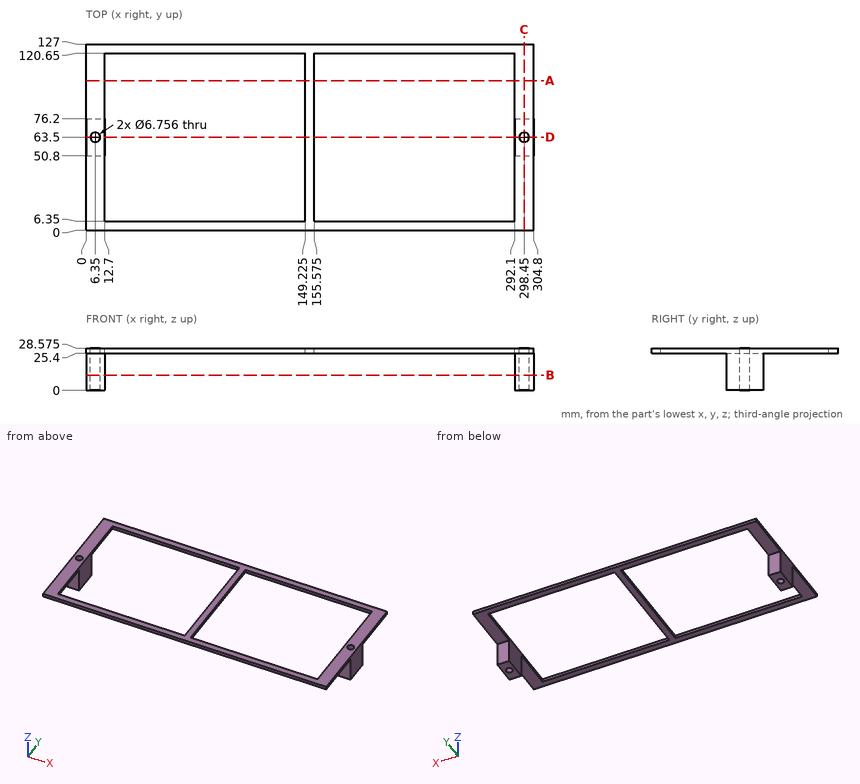
Geometry check sheet. Reference: drawing and pictorial views, mm from the part's lowest x, y, z. Round coordinates to 2 decimals unless told otherwise and drop trailing zeros. Loops run counter-clockwise (first coordinate to the right, second up) from the corner with the lowest first, then second, coordinate; pieces in that order, holes last. Notation, with made-up numbers: (6, -9.5) -> (15, -9.5) arc R17 ccw to (15, -1.5) -> close; hole circle Ø6 at (-10.5, 1.5). An arc over 180 degrees is marked (long way). Use a Markdown table: item, result.
(1) Sectioned sample at D-D (y = 63.5). Enter the section's corners in (x, z) (1 decimal).
Calculated:
| item | result |
|---|---|
| outline | (0, 0) -> (3, 0) -> (3, 28.6) -> (0, 28.6) -> close; (9.7, 0) -> (12.7, 0) -> (12.7, 28.6) -> (9.7, 28.6) -> close; (149.2, 25.4) -> (155.6, 25.4) -> (155.6, 28.6) -> (149.2, 28.6) -> close; (292.1, 0) -> (295.1, 0) -> (295.1, 28.6) -> (292.1, 28.6) -> close; (301.8, 0) -> (304.8, 0) -> (304.8, 28.6) -> (301.8, 28.6) -> close |
(2) Scan lines: probe 1 along X at (y, z) = (63.5, 11); probe 2 along Y at (x, z) = (298.45, 8.5); probe 3 along Y at (x, z) = (180.5, 27.75). Record each from-to range of solid material in increasing order.
Calculated:
| item | result |
|---|---|
| probe 1 | 0 to 2.97, 9.73 to 12.7, 292.1 to 295.07, 301.83 to 304.8 |
| probe 2 | 50.8 to 60.12, 66.88 to 76.2 |
| probe 3 | 0 to 6.35, 120.65 to 127 |
(3) Go/stop test with flat-tipped pins: P1, Ø4, axis at x = 300, z = 18, coming from the +Y side; P2, Ø6.5, axis at x = 298.5, z = 6.5, coming from the -Y side. Record where each tip stops, or that it passes through.
Calculated:
| item | result |
|---|---|
| P1 | y = 76.2 |
| P2 | y = 50.8 |
(4) Sectioned sample at C-C (x = 298.45). Enter the section's corners in (y, z) (1 decimal).
Calculated:
| item | result |
|---|---|
| outline | (0, 25.4) -> (50.8, 25.4) -> (50.8, 0) -> (60.1, 0) -> (60.1, 28.6) -> (0, 28.6) -> close; (66.9, 0) -> (76.2, 0) -> (76.2, 25.4) -> (127, 25.4) -> (127, 28.6) -> (66.9, 28.6) -> close |
(5) Sectioned sample at B-B (z = 10.5). Enter the section's corners in (x, y).
Calculated:
| item | result |
|---|---|
| outline | (0, 50.8) -> (12.7, 50.8) -> (12.7, 76.2) -> (0, 76.2) -> close; (292.1, 50.8) -> (304.8, 50.8) -> (304.8, 76.2) -> (292.1, 76.2) -> close; hole circle Ø6.76 at (6.35, 63.5); hole circle Ø6.76 at (298.45, 63.5) |
(6) Sectioned sample at A-A (y = 102). Enter the section's corners in (x, z) (1 decimal).
Calculated:
| item | result |
|---|---|
| outline | (0, 25.4) -> (12.7, 25.4) -> (12.7, 28.6) -> (0, 28.6) -> close; (149.2, 25.4) -> (155.6, 25.4) -> (155.6, 28.6) -> (149.2, 28.6) -> close; (292.1, 25.4) -> (304.8, 25.4) -> (304.8, 28.6) -> (292.1, 28.6) -> close |
